Here's how the part is built. I have some questions about the finished solid (model axes, mm). Face numbers are marked on the shaded views. A direction names the side the tool comes from. Round coordinates to 2 decimals unless told otherwise and drop trailing zeros. Loops run counter-clockwise (first coordinate to the right, second up) from the corner with the lowest first, then second, coordinate; pieces in that order, holes last. Notation, with made-up numbers: (40, -8) -> (63, -8) arc R21 cw to (63, 24) -> close; hole circle Ø11 at (66.5, 20). An arc over 180 degrees is marked (long way). Use one line per item in the form item = value. Start each with the question number.
Item 1: If we section it at A-A (z = 3.3): Write out the boundary of the cut face in (x, y), then the cut area to 3 significant figures.
Item 2: For the marked faces 4, 5 and 6, which set-ups out of +Z, -Z, +X, -X, +Y, -Y let a thin tool reach every point of the face, with its end or its side?
Item 3: I'm going to push a flat-ended pin straight in: pin 1 Ø1 at (y, z) = (-2, 3.5) entering from -X. Where does the tip first touch, or does it pass through?
Item 4: Thinking about a two-plate mould opening in Y: for the marked faces 1, 2 and 3, which applies, released by +Y, released by -Y, zero draft, split by the parting line, or undercut?
Item 5: If I drill on L1, parallel to Y at x = 0, z = 1.35; L2, parallel to X at y = 0.5, z = 1.9, over which ranges is the centre line in solid material (lowest first)? Write a range as [from, to].
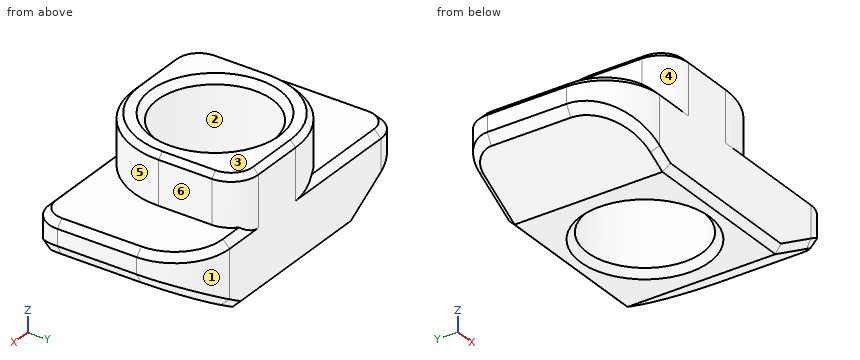
```python
from build123d import *

# Parameters (mm, degrees)
SKETCH_W        = 10.9
SKETCH_H        = 5.9
PAD_DEPTH       = 4.4
SKETCH001_R     = 2.1
HOLE_DEPTH      = 25
SKETCH002_W     = 13.975575
SKETCH002_H     = 8.81763
POCKET_DEPTH    = 1.8
FILLET_R        = 1
FILLET001_R     = 2
FILLET002_R     = 1
POCKET001_DEPTH = 5.901
CHAMFER_SIZE    = 0.25
CHAMFER001_SIZE = 0.2
CHAMFER002_SIZE = 0.25
CHAMFER003_SIZE = 0.25


with BuildPart() as part:
    # Sketch → Pad (new body)
    with BuildSketch(Plane.XY):
        Rectangle(SKETCH_W, SKETCH_H)
    extrude(amount=PAD_DEPTH)

    # Sketch001 (on Face6 of Pad) → Hole (cut)
    with BuildSketch(Plane.XY.offset(4.4)):
        Circle(SKETCH001_R)
    extrude(amount=-HOLE_DEPTH, mode=Mode.SUBTRACT)

    # Sketch002 (on Face5 of Hole) → Pocket (cut)
    with BuildSketch(Plane.XY.offset(4.4)):
        with Locations((0.08922, 0.089121)):
            Rectangle(SKETCH002_W, SKETCH002_H)
        with BuildLine():
            ThreePointArc((0, 2.95), (-2.085965, 2.085965), (-2.95, 0))
            Line((-2.95, 0), (-2.95, -2.95))
            Line((-2.95, -2.95), (0, -2.95))
            ThreePointArc((0, -2.95), (2.085965, -2.085965), (2.95, 0))
            Line((2.95, 2.95), (2.95, 0))
            Line((0, 2.95), (2.95, 2.95))
        make_face(mode=Mode.SUBTRACT)
    extrude(amount=-POCKET_DEPTH, mode=Mode.SUBTRACT)

    # Fillet
    fillet_edges = [part.edges().sort_by_distance(p)[0] for p in [
        (2.95, 2.95, 3.5),
        (-2.95, -2.95, 3.5),
    ]]
    fillet(fillet_edges, radius=FILLET_R)

    # Fillet001
    fillet001_edges = [part.edges().sort_by_distance(p)[0] for p in [
        (5.45, 2.95, 1.3),
        (-5.45, -2.95, 1.3),
    ]]
    fillet(fillet001_edges, radius=FILLET001_R)

    # Fillet002
    fillet002_edges = [part.edges().sort_by_distance(p)[0] for p in [
        (5.45, -2.95, 1.3),
        (-5.45, 2.95, 1.3),
    ]]
    fillet(fillet002_edges, radius=FILLET002_R)

    # Sketch003 (on Face5 of Fillet002) → Pocket001 (cut, through all)
    with BuildSketch(Plane.XZ.offset(2.95)):
        Polygon((-5.45, 1.5), (-2.95, 0), (-5.45, 0), align=None)
        Polygon((5.45, 1.5), (5.45, 0), (2.95, 0), align=None)
    extrude(amount=-POCKET001_DEPTH, mode=Mode.SUBTRACT)

    # Chamfer
    chamfer_edges = [part.edges().sort_by_distance(p)[0] for p in [
        (-2.1, 0, 0),
        (-2.1, 0, 4.4),
    ]]
    chamfer(chamfer_edges, length=CHAMFER_SIZE)

    # Chamfer001
    chamfer001_edges = [part.edges().sort_by_distance(p)[0] for p in [
        (-2.95, -0.975, 4.4),
    ]]
    chamfer(chamfer001_edges, length=CHAMFER001_SIZE)

    # Chamfer002
    chamfer002_edges = [part.edges().sort_by_distance(p)[0] for p in [
        (0, -2.95, 0),
        (3.7, -2.95, 0.45),
        (-3.2, -2.95, 0.15),
        (0, 2.95, 0),
    ]]
    chamfer(chamfer002_edges, length=CHAMFER002_SIZE)

    # Chamfer003
    chamfer003_edges = [part.edges().sort_by_distance(p)[0] for p in [
        (-4.864214, -2.364214, 2.6),
        (2.225, -2.95, 2.6),
    ]]
    chamfer(chamfer003_edges, length=CHAMFER003_SIZE)


solid = part.part
```
Values found:
q1.outline = (-2.95, -1.95) arc R1 ccw to (-1.95, -2.95) -> (0, -2.95) arc R2.95 ccw to (2.95, 0) -> (2.95, 1.95) arc R1 ccw to (1.95, 2.95) -> (0, 2.95) arc R2.95 ccw to (-2.95, 0) -> close; hole circle Ø4.2 at (0, 0)
q1.area = 16.8 mm2
q2.face_4 = +Z, -X, -Y
q2.face_5 = +Z, +X, -Y
q2.face_6 = +Z, +X, +Y, -Y
q3.pin_1 = -2.95
q4.face_1 = released by +Y
q4.face_2 = undercut
q4.face_3 = zero draft
q5.L1 = [-2.95, -2.1], [2.1, 2.95]
q5.L2 = [-5.45, -2.04], [2.04, 5.45]
